Input: part model. Units: mm. Frame: model coordinates. Face numbers are marked on the shaded views. A direction names the side the tool comes from. Round coordinates to 2 decimals unless told otherwise and drop trailing zeros. Loops run counter-clockwise (first coordinate to the right, second up) from the corner with the lowest first, then second, coordinate; pieces in that order, holes last. Notation, with made-up numbers: M 21,27 L 72,27 A13 ccw 72,51 Z; hole C 61,-34.75 d2. An arc over 180 degrees is marked long. Return JSON: item names as keys, results as strings. Group by question number.
1) Section A-A (z = -5.5). Output: boundary loops of the cut face in (x, y), plus the area to 3 significant figures.
2) Section B-B (x = -39). Output: boundary loops of the cut face in (y, z).
3) Section C-C (z = -10). Output: boundary loops of the cut face in (x, y).
4) Material intervals for line 1 (X direction, y = 2.5, z = -5.5); line 2 (X direction, y = 18.25, z = -9); line 3 (X direction, y = 15, z = -21.5), sorted ascending. Write a range as from..to.
5) Section D-D (x = -4). Output: boundary loops of the cut face in (y, z), plus the area to 3 significant figures.
6) Contact query for flat-ended pins moving along their axis: P1, Ø8, axis at x = -39, z = -5.5, coming from the -Y side; P2, Ø1, axis at x = 26.5, z = -32.5, coming from the -Y side; P3, Ø10.5, axis at x = 39, z = -14.5, coming from the +Y side; P4, Ø6, axis at y = 13, z = -14.5, coming from the +X side. Output: stop coordinate, or through.
7) Mould query, pull axis X, two halves, no side actions, for the marked faces 1, 2, 3 and 4. Classes: +X half, -X half, draft (parallel to the pull), parting line (faces both ways), or undercut.
8) Access query for the marked faces 5 and 6. Directions: +Z, -Z, +X, -X, +Y, -Y. A direction counts if a zero-diameter tool reaches every point of the face in a straight line with its end or side. Return the directions, or none.
from build123d import *

# Parameters (mm, degrees)
SKETCH_13_W         = 90
SKETCH_13_H         = 40
EXTRUDE_8_DEPTH     = 25.3
SKETCH_15_W         = 66
SKETCH_15_H         = 40
CUT_EXTRUDE_3_DEPTH = 1
SKETCH_17_W         = 12
SKETCH_17_H         = 21
CUT_EXTRUDE_4_DEPTH = 40
EXTRUDE_10_DEPTH    = 12
FILLET_1_R          = 1
FILLET_2_R          = 1
FILLET_3_R          = 1
CUT_EXTRUDE_5_REACH = 65.765
SKETCH_22_R         = 3.1


with BuildPart() as part:
    # 草图13 → 凸台-拉伸8 (new body)
    with BuildSketch(Plane(origin=(0, 0, 0), x_dir=(1, 0, 0), z_dir=(0, 1, 0))):
        with Locations((0, 20)):
            Rectangle(SKETCH_13_W, SKETCH_13_H)
    extrude(amount=EXTRUDE_8_DEPTH)

    # 草图15 → 切除-拉伸3 (cut)
    with BuildSketch(Plane.XZ):
        with Locations((0, -20)):
            Rectangle(SKETCH_15_W, SKETCH_15_H)
    extrude(amount=-CUT_EXTRUDE_3_DEPTH, mode=Mode.SUBTRACT)

    # 草图17 → 切除-拉伸4 (cut)
    with BuildSketch(Plane.XY):
        with Locations((-39, 14.8)):
            Rectangle(SKETCH_17_W, SKETCH_17_H)
        with Locations((39, 14.8)):
            Rectangle(SKETCH_17_W, SKETCH_17_H)
    extrude(amount=-CUT_EXTRUDE_4_DEPTH, mode=Mode.SUBTRACT)

    # 草图19 → 凸台-拉伸10 (add)
    with BuildSketch(Plane.ZY.offset(33)):
        Polygon((-13.58148117, 18.169722386), (-20, 14.8), (-13.778047619, 11.533475), (-12.839009712, 17.571921973), align=None)
        Polygon((-25.98104999, 19.61563852), (-26.221952381, 18.066525), (-20, 14.8), (-13.58148117, 18.169722386), (-18.820059701, 22.387560492), align=None)
        Polygon((-20, 14.8), (-26.221952381, 18.066525), (-27.160990288, 12.028078027), (-26.41851883, 11.430277614), align=None)
        Polygon((-13.778047619, 11.533475), (-20, 14.8), (-26.41851883, 11.430277614), (-21.179940299, 7.212439508), (-14.01895001, 9.98436148), align=None)
    extrude(amount=EXTRUDE_10_DEPTH)

    # 圆角1
    fillet_1_edges = [part.edges().sort_by_distance(p)[0] for p in [
        (0, 25.3, 0),
    ]]
    fillet(fillet_1_edges, radius=FILLET_1_R)

    # 圆角2
    fillet_2_edges = [part.edges().sort_by_distance(p)[0] for p in [
        (0, 25.3, -40),
        (-33, 25.3, -20.5),
        (-33, 14.3, 0),
        (33, 14.3, 0),
        (33, 25.3, -20.5),
        (33, 25.007106781, -0.292893219),
        (-33, 25.007106781, -0.292893219),
    ]]
    fillet(fillet_2_edges, radius=FILLET_2_R)

    # 圆角3
    fillet_3_edges = [part.edges().sort_by_distance(p)[0] for p in [
        (-45, 21.001599506, -22.400554846),
        (-39, 22.387560492, -18.820059701),
        (-45, 19.979741232, -15.829534706),
        (-39, 17.571921973, -12.839009712),
        (-45, 13.778141726, -13.428979861),
        (-39, 9.98436148, -14.01895001),
        (-45, 8.598400494, -17.599445154),
        (-39, 7.212439508, -21.179940299),
        (-45, 9.620258768, -24.170465294),
        (-39, 12.028078027, -27.160990288),
        (-45, 15.821858274, -26.571020139),
        (-39, 19.61563852, -25.98104999),
    ]]
    fillet(fillet_3_edges, radius=FILLET_3_R)

    # 草图22 → 切除-拉伸5 (cut, up to next)
    with BuildSketch(Plane(origin=(0, 4.3, 0), x_dir=(1, 0, 0), z_dir=(0, 1, 0)), mode=Mode.PRIVATE) as cut_extrude_5_sk1:
        with Locations(Location((-39, 5.5, 0), (0, 0, 270))):
            Circle(SKETCH_22_R)
    cut_extrude_5_tool1 = extrude(cut_extrude_5_sk1.sketch, amount=-CUT_EXTRUDE_5_REACH, mode=Mode.PRIVATE) & part.part
    # 草图22 → 切除-拉伸5 (cut, up to next)
    with BuildSketch(Plane(origin=(0, 4.3, 0), x_dir=(1, 0, 0), z_dir=(0, 1, 0)), mode=Mode.PRIVATE) as cut_extrude_5_sk2:
        with Locations(Location((39, 5.5, 0), (0, 0, 270))):
            Circle(SKETCH_22_R)
    cut_extrude_5_tool2 = extrude(cut_extrude_5_sk2.sketch, amount=-CUT_EXTRUDE_5_REACH, mode=Mode.PRIVATE) & part.part
    # 草图22 → 切除-拉伸5 (cut, up to next)
    with BuildSketch(Plane(origin=(0, 4.3, 0), x_dir=(1, 0, 0), z_dir=(0, 1, 0)), mode=Mode.PRIVATE) as cut_extrude_5_sk3:
        with Locations(Location((39, 34.5, 0), (0, 0, 270))):
            Circle(SKETCH_22_R)
    cut_extrude_5_tool3 = extrude(cut_extrude_5_sk3.sketch, amount=-CUT_EXTRUDE_5_REACH, mode=Mode.PRIVATE) & part.part
    # 草图22 → 切除-拉伸5 (cut, up to next)
    with BuildSketch(Plane(origin=(0, 4.3, 0), x_dir=(1, 0, 0), z_dir=(0, 1, 0)), mode=Mode.PRIVATE) as cut_extrude_5_sk4:
        with Locations(Location((-39, 34.5, 0), (0, 0, 270))):
            Circle(SKETCH_22_R)
    cut_extrude_5_tool4 = extrude(cut_extrude_5_sk4.sketch, amount=-CUT_EXTRUDE_5_REACH, mode=Mode.PRIVATE) & part.part
    add(cut_extrude_5_tool1.solids().sort_by_distance((-39, 4.3, -5.5))[0], mode=Mode.SUBTRACT)
    add(cut_extrude_5_tool2.solids().sort_by_distance((39, 4.3, -5.5))[0], mode=Mode.SUBTRACT)
    add(cut_extrude_5_tool3.solids().sort_by_distance((39, 4.3, -34.5))[0], mode=Mode.SUBTRACT)
    add(cut_extrude_5_tool4.solids().sort_by_distance((-39, 4.3, -34.5))[0], mode=Mode.SUBTRACT)


solid = part.part
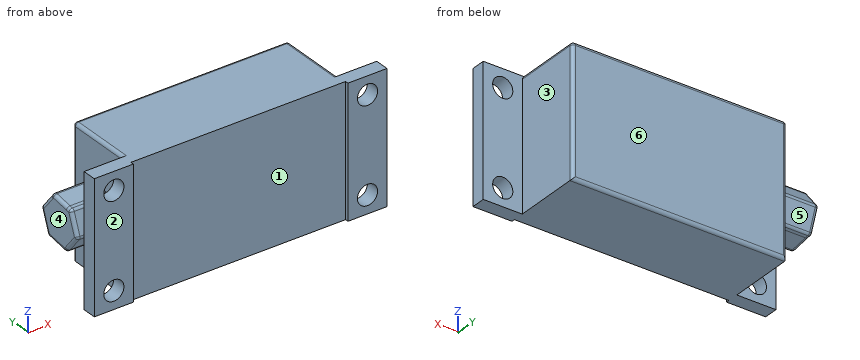
Returned:
{
 "1": {"outline": "M -45,0 L -42.1,0 L -42.1,4.3 L -45,4.3 Z; M -35.9,0 L -33,0 L -33,1 L 33,1 L 33,0 L 35.9,0 L 35.9,4.3 L 33,4.3 L 33,24.3 A1 ccw 32,25.3 L -32,25.3 A1 ccw -33,24.3 L -33,4.3 L -35.9,4.3 Z; M 42.1,0 L 45,0 L 45,4.3 L 42.1,4.3 Z", "area": "1,650 mm^2"},
 "2": {"outline": "M 0,-40 L 4.3,-40 L 4.3,-37.6 L 0,-37.6 Z; M 0,-31.4 L 4.3,-31.4 L 4.3,-8.6 L 0,-8.6 Z; M 0,-2.4 L 4.3,-2.4 L 4.3,0 L 0,0 Z; M 7.42,-20.64 A1 ccw 7.57,-21.63 L 11.67,-26.71 A1 ccw 12.6,-27.07 L 19.05,-26.07 A1 ccw 19.82,-25.44 L 22.18,-19.36 A1 ccw 22.03,-18.37 L 17.93,-13.29 A1 ccw 17,-12.93 L 10.55,-13.93 A1 ccw 9.78,-14.56 Z"},
 "3": {"outline": "M -45,0 L -33,0 L -33,1 L 33,1 L 33,0 L 45,0 L 45,4.3 L 33,4.3 L 33,24.3 A1 ccw 32,25.3 L -32,25.3 A1 ccw -33,24.3 L -33,4.3 L -45,4.3 Z"},
 "4": {"line 1": "x = -45..-42.1, -35.9..35.9, 42.1..45", "line 2": "x = -33..33", "line 3": "x = -45..33"},
 "5": {"outline": "M 1,-40 L 24.3,-40 A1 ccw 25.3,-39 L 25.3,-1 A1 ccw 24.3,0 L 1,0 Z", "area": "972 mm^2"},
 "6": {"P1": "stops at y = 0", "P2": "stops at y = 1", "P3": "stops at y = 4.3", "P4": "stops at x = 33"},
 "7": {"face 1": "undercut", "face 2": "draft", "face 3": "+X half", "face 4": "-X half"},
 "8": {"face 5": "-Z, -X, +Y", "face 6": "+Z, -Z, +X, -X, +Y"}
}
